Model file for the job. Use its own axes, mm. A direction names the side the tool comes from. Round coordinates to 2 decimals unless told otherwise and drop trailing zeros. Loops run counter-clockwise (first coordinate to the right, second up) from the corner with the lowest first, then second, coordinate; pieces in that order, holes last.
from build123d import *

# Parameters (mm, degrees)
BOSS_EXTRU_1_DEPTH = 5.125
ESQUISSE2_R        = 2.5
BOSS_EXTRU_2_DEPTH = 15
ESQUISSE3_R        = 2.5
BOSS_EXTRU_3_DEPTH = 10


with BuildPart() as part:
    # Esquisse1 → Boss.-Extru.1 (new body, symmetric)
    with BuildSketch(Plane.XY):
        with BuildLine():
            Line((-28.790189362, 6.603053435), (145.209810638, 6.603053435))
            ThreePointArc((145.209810638, 6.603053435), (150.209810638, 1.603053435), (145.209810638, -3.396946565))
            Line((145.209810638, -3.396946565), (-28.790189362, -3.396946565))
            ThreePointArc((-28.790189362, -3.396946565), (-33.790189362, 1.603053435), (-28.790189362, 6.603053435))
        make_face()
    extrude(amount=BOSS_EXTRU_1_DEPTH, both=True)

    # Esquisse2 → Boss.-Extru.2 (add)
    with BuildSketch(Plane.XY):
        with Locations((-28.790189362, 1.603053435)):
            Circle(ESQUISSE2_R)
    extrude(amount=BOSS_EXTRU_2_DEPTH)

    # Esquisse3 → Boss.-Extru.3 (add)
    with BuildSketch(Plane.XY):
        with Locations((145.209810638, 1.603053435)):
            Circle(ESQUISSE3_R)
    extrude(amount=-BOSS_EXTRU_3_DEPTH)


solid = part.part
Q1. Slice it at A-A on x = 131.5. Give the cut face in (y, z) (3 decimals), plus the area to 4 significant figures.
Q2. Flat gauge pins, fed straight in: P1, Ø1.5, axis at x = 10, y = 0.5, coming from the -Z side (3 decimals); P2, Ø5, axis at x = -1, y = 4, coming from the +Z side (3 decimals); P3, Ø6, axis at y = 0, z = 4.5, coming from the +X side; P4, Ø1.5, axis at y = 1, z = -7.5, coming from the -X side. Where does each tip first touch, or does it go through?
Q3. Probe line 1 (Z direction, x = -4.5, y = -1) (3 decimals); line 2 (X direction, y = 1.75, z = 8.25); line 3 (X direction, y = 5, z = -1.25). List the from-to ranges inside material, lowest first.
Q4. Tool access for faces 1 (the face through (147.5, 0.6, -7.5)), 2 (the face through (-30.633, 3.293, 9.993)), 3 (the face through (145, 2, -10)): list every direction of +Z, -Z, +X, -X, +Y, -Y with a clear straight run to the whole face (end or side of a thin tool).
Q5. Slice it at B-B on z = -7.75. Give the cut face in (x, y), plus the area to 3 significant figures.
Reply:
1. outline: (-3.397, -5.125) - (6.603, -5.125) - (6.603, 5.125) - (-3.397, 5.125) - close
1. area: 102.5 mm2
2. P1: stops at z = -5.125
2. P2: stops at z = 5.125
2. P3: stops at x = 150.21
2. P4: stops at x = 142.71
3. line 1: z = -5.125 to 5.125
3. line 2: x = -31.29 to -26.29
3. line 3: x = -32.46 to 148.88
4. face 1: -Z
4. face 2: +Z
4. face 3: -Z, +X, -X, +Y, -Y
5. outline: circle Ø5 at (145.21, 1.6)
5. area: 19.6 mm2
